Autodesk Inventor part; units mm, degrees
ref_plane "YZ Plane" through (0, 0, 0) normal (1, 0, 0) x (0, 1, 0)
ref_plane "XZ Plane" through (0, 0, 0) normal (0, 1, 0) x (-1, 0, 0)
ref_plane "XY Plane" through (0, 0, 0) normal (0, 0, 1) x (1, 0, 0)
sketch "Sketch1" plane through (0, 0, 0) normal (0, 1, 0) x (-1, 0, 0)
  circle A0 centre (0, 0) radius 50
  circle A1 centre (0, 0) radius 6.25
  dimension "d0" = 100
  dimension "d1" = 12.5
extrude "Extrusion1" add sketch "Sketch1" along normal blind 5
sketch "Sketch2" plane through (0, 5, 0) normal (0, 1, 0) x (1, 0, 0)
  line L0 (9.75, 0) -> (4.875, -8.4437)
  line L1 (4.875, -8.4437) -> (-4.875, -8.4437)
  line L2 (-4.875, -8.4437) -> (-9.75, 0)
  line L3 (-9.75, 0) -> (-4.875, 8.4437)
  line L4 (-4.875, 8.4437) -> (4.875, 8.4437)
  line L5 (4.875, 8.4437) -> (9.75, 0)
  line L6 (0, 0) -> (0, 50) construction
  circle A0 centre (0, 0) radius 50 construction
  line L7 (0, 0) -> (-50, 0) construction
  circle A1 centre (0, 0) radius 15
  dimension "d4" = 19.5
  dimension "d5" = 30
extrude "Extrusion2" add sketch "Sketch2" along normal blind 10
sketch "Sketch3" plane through (0, 5, 0) normal (0, 1, 0) x (1, 0, 0)
  circle A0 centre (0, 0) radius 50
  circle A1 centre (0, 0) radius 47.5
  dimension "d8" = 95
extrude "Extrusion3" add sketch "Sketch3" along normal blind 5
sketch "Sketch4" plane through (0, 10, 0) normal (0, 1, 0) x (1, 0, 0)
  circle A0 centre (0, 0) radius 15
  circle A1 centre (0, 0) radius 50
extrude "Extrusion4" add sketch "Sketch4" along normal blind 5
sketch "Sketch5" plane through (0, 0, 0) normal (0, -1, 0) x (1, 0, 0)
  circle A0 centre (0, 0) radius 6.25 construction
  line L0 (0, 0) -> (0, -50) construction
  circle A1 centre (0, 0) radius 50 construction
  line L1 (0, 0) -> (50, 0) construction
  circle A2 centre (25, -25) radius 10
  circle A3 centre (-25, -25) radius 10
  circle A4 centre (25, 25) radius 10
  circle A5 centre (-25, 25) radius 10
  dimension "d13" = 20
  dimension "d14" = 25
  dimension "d15" = 25
extrude "Extrusion5" add sketch "Sketch5" along normal blind 20
draft "FaceDraft1" angle 15 pull direction (0, -1, 0) faces at (34.8705, -13.3333, -26.6041) fixed edges at (15, 0, -25)
draft "FaceDraft3" angle 15 pull direction (0, -1, 0) faces at (-15.1295, -13.3333, -26.6041) fixed edges at (-35, 0, -25)
draft "FaceDraft4" angle 15 pull direction (0, -1, 0) faces at (34.8705, -13.3333, 23.3959) fixed edges at (15, 0, 25)
draft "FaceDraft5" angle 15 pull direction (0, -1, 0) faces at (-15.1295, -13.3333, 23.3959) fixed edges at (-35, 0, 25)
chamfer "Chamfer1" distance 2 angle 45 1 edges at (-50, 15, 0)
chamfer "Chamfer2" distance 2 angle 45 1 edges at (50, 0, 0)
properties part number "ground_support_2"
The model under review builds one solid part; all positions refer to its coordinate system, in mm. A direction names the side the tool comes from. Round coordinates to 2 decimals unless told otherwise and drop trailing zeros. Loops run counter-clockwise (first coordinate to the right, second up) from the corner with the lowest first, then second, coordinate; pieces in that order, holes last. Notation, with made-up numbers: M 27.5,70.5 L 65.5,70.5 A14 ccw 65.5,84.5 Z; hole C 35,-9 d2. An arc over 180 degrees is marked long. Answer as CSV lines item,"result". Start each with the question number.
Item 1: Consider section B-B (x = 0). Write out the cut boundary in (y, z).
Item 2: Consider section C-C (y = -6.5). Write out the cut boundary in (x, z), then the cut area to 3 significant figures.
Item 3: Wall thickness on line 1 (Z direction, x = 0, y = 6.15); line 2 (Z direction, x = 0, y = 3.6); line 3 (Y direction, x = 30, z = 15): over which ranges is each line inside the solid? List them lowest first. Write a range as [from, to].
Item 4: Consider section A-A (y = 8.5). Write out the cut boundary in (x, z) (3 decimals).
Item 5: Mouldability with a two-part tool opening along X and no side actions: class faces 5 (the face through (-6.4, 5, 0.1)), 6 (the face through (25, -20, 25)), 7 (the face through (-44.46, 0.13, -18.43)) as released by +X, released by -X, zero draft, split by the parting line, or undercut.
Item 6: Insertion check: P1, Ø8, axis at x = -30.5, y = -2.5, coming from the -Z side (3 decimals); P2, Ø10, axis at x = -32.5, z = -10.5, coming from the -Y side; P3, Ø10, axis at y = 5.5, z = 15, coming from the -X side. Each pin has a flat end and moves straight along its axis. Give the tip position at first contact, or say it passes through.
Item 7: For faces 1 (the face through (0, 10, 8.444)), 2 (the face through (25, -20, -25)), 3 (the face through (-10.3, 7.46, -46.37)), 4 (the face through (1, 0, -10)), list the 3-axis set-ups (+Z, -Z, +X, -X, +Y, -Y) from which the entire face can be reached by the end or side of a thin tool; tool diameter is ignored.
Answer:
1,outline,"M 0,-48 L 2,-50 L 13,-50 L 15,-48 L 15,-8.44 L 5,-8.44 L 5,-6.25 L 0,-6.25 Z; M 0,6.25 L 5,6.25 L 5,8.44 L 15,8.44 L 15,48 L 13,50 L 2,50 L 0,48 Z; hole M 5,-47.5 L 10,-47.5 L 10,-15 L 5,-15 Z; hole M 5,15 L 10,15 L 10,47.5 L 5,47.5 Z"
2,outline,"C -25,-25 d16.52; C -25,25 d16.52; C 25,-25 d16.52; C 25,25 d16.52"
2,area,"857 mm^2"
3,line 1,"z = [-50, -47.5], [-15, -8.44], [8.44, 15], [47.5, 50]"
3,line 2,"z = [-50, -6.25], [6.25, 50]"
3,line 3,"y = [0, 5], [10, 15]"
4,outline,"C 0,0 d100; C 0,0 d30; hole C 0,0 d95; hole M -9.75,0 L -4.875,-8.444 L 4.875,-8.444 L 9.75,0 L 4.875,8.444 L -4.875,8.444 Z"
5,face 5,"undercut"
5,face 6,"zero draft"
5,face 7,"split by the parting line"
6,P1,"stops at z = -39.815"
6,P2,"stops at y = 0"
6,P3,"stops at x = -48.99"
7,face 1,"+Y"
7,face 2,"+Z, -Z, +X, -X, -Y"
7,face 3,"none"
7,face 4,"-Y"
